Work out the finished part from the listing and answer in its coordinate system (mm). Give positions to 0.01 mm unless a question says otherwise; leave off trailing zeros. Order: outer loops, then holes, each group sorted by start corner. A loop starts at its lowest first (then second) coordinate and runs counter-clockwise, first axis right, second up. Notation, with made-up numbers: M 24,89 L 47,89 A24 ccw 47,113 Z; hole C -8,88 d10. An arc over 180 degrees is marked long. One line per item, written item: value.
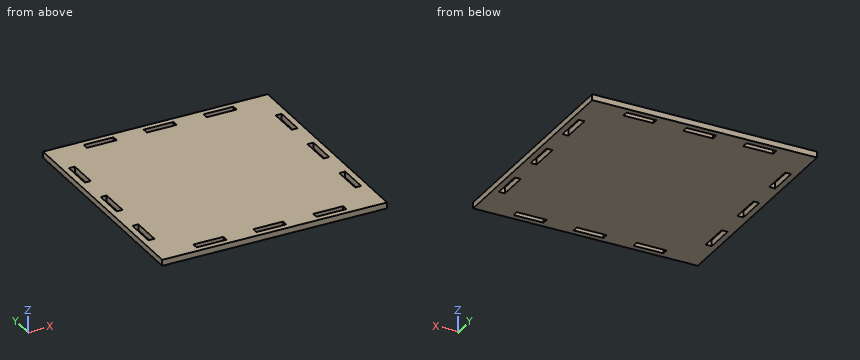
from build123d import *

# Parameters (mm, degrees)
F0_W     = 150
F0_H     = 150
F1_DEPTH = 4


with BuildPart() as f1:
    # F0 (on Top) → F1 (new body)
    with BuildSketch(Plane.XY):
        Rectangle(F0_W, F0_H)
        Polygon((-30, -71), (-40, -71), (-50, -71), (-50, -67), (-40, -67), (-30, -67), align=None, mode=Mode.SUBTRACT)
        Polygon((-71, -30), (-67, -30), (-67, -50), (-71, -50), (-71, -40), align=None, mode=Mode.SUBTRACT)
        Polygon((-10, -71), (-10, -67), (0, -67), (10, -67), (10, -71), (0, -71), align=None, mode=Mode.SUBTRACT)
        Polygon((50, -71), (40, -71), (30, -71), (30, -67), (40, -67), (50, -67), align=None, mode=Mode.SUBTRACT)
        Polygon((71, -50), (67, -50), (67, -30), (71, -30), (71, -40), align=None, mode=Mode.SUBTRACT)
        Polygon((-71, -10), (-71, 0), (-71, 10), (-67, 10), (-67, 0), (-67, -10), align=None, mode=Mode.SUBTRACT)
        Polygon((-71, 50), (-67, 50), (-67, 30), (-71, 30), (-71, 40), align=None, mode=Mode.SUBTRACT)
        Polygon((-30, 71), (-30, 67), (-40, 67), (-50, 67), (-50, 71), (-40, 71), align=None, mode=Mode.SUBTRACT)
        Polygon((71, 0), (71, -10), (67, -10), (67, 10), (71, 10), align=None, mode=Mode.SUBTRACT)
        Polygon((-10, 71), (0, 71), (10, 71), (10, 67), (0, 67), (-10, 67), align=None, mode=Mode.SUBTRACT)
        Polygon((71, 30), (67, 30), (67, 50), (71, 50), (71, 40), align=None, mode=Mode.SUBTRACT)
        Polygon((30, 71), (40, 71), (50, 71), (50, 67), (40, 67), (30, 67), align=None, mode=Mode.SUBTRACT)
    extrude(amount=F1_DEPTH)


solid = f1.part
(1) Given P1, Ø3, axis at x = -9.5, y = -58.5, coming from the -Z side, flat-ended and moving along its own axis, determine where the tip first touches the part or whether it passes through.
Findings:
P1: stops at z = 0
(2) Section A-A, the plane x = 42.5 is taken. Give the vertices of the cut face in (y, z).
Findings:
outline: M -75,0 L -71,0 L -71,4 L -75,4 Z; M -67,0 L 67,0 L 67,4 L -67,4 Z; M 71,0 L 75,0 L 75,4 L 71,4 Z
(3) Section C-C, the plane z = 2 is taken. Give the number of separate pieces and of enclosed holes in the cut face, then the cut area to 3 significant figures.
Findings:
separate pieces: 1
enclosed holes: 12
area: 21,500 mm^2
(4) Find the intervals of material crossed by probe 1 along Y at (x, z) = (40, 2.3), in increasing order. Write a range as from..to.
Findings:
probe 1: y = -75..-71, -67..67, 71..75
